Build history of the part. All positions in model axes, mm. Face numbers are marked on the shaded views. A direction names the side the tool comes from. Coordinates: 2 decimals unless noted, no trailing zeros. Order: outer loops, then holes, each group sorted by start corner. A loop starts at its lowest first (then second) coordinate and runs counter-clockwise, first axis right, second up. Notation, with made-up numbers: (69, 33) - (83, 33) arc R9 cw to (83, 42) - close; hole circle Ø10 at (8, 79). An arc over 180 degrees is marked (long way). Return JSON: item names as keys, results as strings.
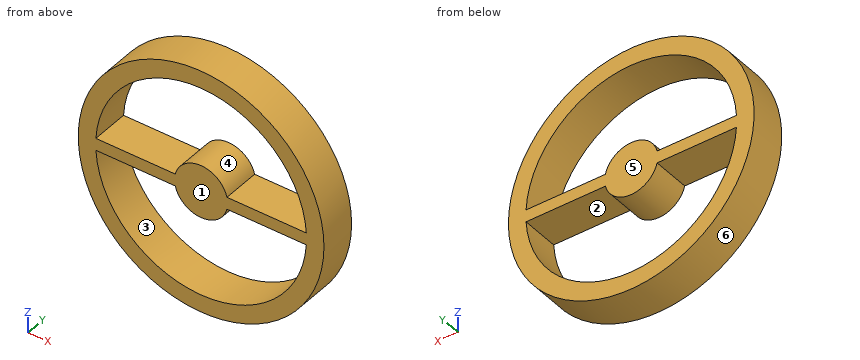
from build123d import *

# Parameters (mm, degrees)
F0_R     = 10.3601879012
F1_DEPTH = 3.175
F2_R     = 10.3601879012
F3_DEPTH = 3.175


with BuildPart() as f1:
    # F0 (on Front) → F1 (new body)
    with BuildSketch(Plane.XZ):
        Circle(F0_R)
        with BuildLine():
            ThreePointArc((9.5114533333, 0.5078193457), (9.521612731, 0.254), (9.525, 0))
            ThreePointArc((9.525, 0), (9.5215246826, -0.2572794566), (9.5111012664, -0.5143711699))
            ThreePointArc((9.5111012664, -0.5143711699), (0, -9.525), (-9.5111012664, -0.5143711699))
            ThreePointArc((-9.5111012664, -0.5143711699), (-9.524999435, -0.0032806383), (-9.5114533333, 0.5078193457))
            ThreePointArc((-9.5114533333, 0.5078193457), (0, 9.525), (9.5114533333, 0.5078193457))
        make_face(mode=Mode.SUBTRACT)
        with BuildLine():
            Line((-2.1784585047, 0.5078193457), (-9.5114533333, 0.5078193457))
            ThreePointArc((-9.5114533333, 0.5078193457), (-9.524999435, -0.0032806383), (-9.5111012664, -0.5143711699))
            Line((-9.5111012664, -0.5143711699), (-2.1769208171, -0.5143711699))
            ThreePointArc((-2.1769208171, -0.5143711699), (-2.2368617797, -0.0033649251), (-2.1784585047, 0.5078193457))
        make_face()
        with BuildLine():
            ThreePointArc((2.2368643107, 0), (2.222214889, 0.2555835118), (2.1784585047, 0.5078193457))
            ThreePointArc((2.1784585047, 0.5078193457), (0, 2.2368643107), (-2.1784585047, 0.5078193457))
            ThreePointArc((-2.1784585047, 0.5078193457), (-2.2368617797, -0.0033649251), (-2.1769208171, -0.5143711699))
            ThreePointArc((-2.1769208171, -0.5143711699), (0, -2.2368643107), (2.1769208171, -0.5143711699))
            ThreePointArc((2.1769208171, -0.5143711699), (2.2218278992, -0.2589261105), (2.2368643107, 0))
        make_face()
        with BuildLine():
            ThreePointArc((9.5111012664, -0.5143711699), (9.5215246826, -0.2572794566), (9.525, 0))
            ThreePointArc((9.525, 0), (9.521612731, 0.254), (9.5114533333, 0.5078193457))
            Line((9.5114533333, 0.5078193457), (2.1784585047, 0.5078193457))
            ThreePointArc((2.1784585047, 0.5078193457), (2.222214889, 0.2555835118), (2.2368643107, 0))
            ThreePointArc((2.2368643107, 0), (2.2218278992, -0.2589261105), (2.1769208171, -0.5143711699))
            Line((2.1769208171, -0.5143711699), (9.5111012664, -0.5143711699))
        make_face()
    extrude(amount=F1_DEPTH)

    # F2 (on face) → F3 (join)
    with BuildSketch(Plane.XZ.offset(3.175)):
        Circle(F2_R)
        with BuildLine():
            ThreePointArc((8.8731253784, 0.5078193457), (8.8840143878, 0.2540134389), (8.8876450463, 0))
            ThreePointArc((8.8876450463, 0), (8.8839199998, -0.2572934234), (8.872747983, -0.5143711699))
            Line((8.872747983, -0.5143711699), (9.5111012664, -0.5143711699))
            ThreePointArc((9.5111012664, -0.5143711699), (0, -9.525), (-9.5111012664, -0.5143711699))
            Line((-9.5111012664, -0.5143711699), (-8.872747983, -0.5143711699))
            ThreePointArc((-8.872747983, -0.5143711699), (-8.8876444406, -0.0032813423), (-8.8731253784, 0.5078193457))
            Line((-8.8731253784, 0.5078193457), (-9.5114533333, 0.5078193457))
            ThreePointArc((-9.5114533333, 0.5078193457), (0, 9.525), (9.5114533333, 0.5078193457))
            Line((9.5114533333, 0.5078193457), (8.8731253784, 0.5078193457))
        make_face(mode=Mode.SUBTRACT)
        with BuildLine():
            ThreePointArc((-8.8731253784, 0.5078193457), (0, 8.8876450463), (8.8731253784, 0.5078193457))
            Line((8.8731253784, 0.5078193457), (9.5114533333, 0.5078193457))
            ThreePointArc((9.5114533333, 0.5078193457), (0, 9.525), (-9.5114533333, 0.5078193457))
            Line((-9.5114533333, 0.5078193457), (-8.8731253784, 0.5078193457))
        make_face()
        with BuildLine():
            Line((9.5111012664, -0.5143711699), (8.872747983, -0.5143711699))
            ThreePointArc((8.872747983, -0.5143711699), (0, -8.8876450463), (-8.872747983, -0.5143711699))
            Line((-8.872747983, -0.5143711699), (-9.5111012664, -0.5143711699))
            ThreePointArc((-9.5111012664, -0.5143711699), (0, -9.525), (9.5111012664, -0.5143711699))
        make_face()
    extrude(amount=-F3_DEPTH)


solid = f1.part
1. Cut at A-A on x = 0. Give the cut face in (y, z) (3 decimals).
Check values:
{"outline": "(-3.175, -10.36) - (0, -10.36) - (0, -8.888) - (-3.175, -8.888) - close; (-3.175, -2.237) - (0, -2.237) - (0, 2.237) - (-3.175, 2.237) - close; (-3.175, 8.888) - (0, 8.888) - (0, 10.36) - (-3.175, 10.36) - close"}
2. Drop flat-ended pins along their axis: pin 1 (1.6 mm diameter, centred on x = -4.5, y = -2, fed in from +Z); pin 2 (1.5 mm diameter, centred on y = -3, z = 2.5, fed in from +X); pin 3 (2 mm diameter, centred on x = -2.5, z = 1.5, fed in from +Y); pin 4 (1 mm diameter, centred on x = 6, y = -2, fed in from -Z). Give the stop position or say it passes through.
Check values:
{"pin 1": "z = 9.68", "pin 2": "x = 10.21", "pin 3": "y = 0", "pin 4": "z = -8.78"}
3. Tool access for the marked faces 1 and 2: list every direction of +Z, -Z, +X, -X, +Y, -Y with a clear straight run to the whole face (end or side of a thin tool).
Check values:
{"face 1": "+Z, -Z, +X, -X, -Y", "face 2": "+Y, -Y"}
4. Cut at C-C on z = -4.75. Give the cut face in (x, y) (3 decimals).
Check values:
{"outline": "(-9.207, -3.175) - (-7.512, -3.175) - (-7.512, 0) - (-9.207, 0) - close; (7.512, -3.175) - (9.207, -3.175) - (9.207, 0) - (7.512, 0) - close"}
5. Cut at D-D on z = 3.5. Give the cut face in (x, y) (3 decimals), plus the area to 3 significant figures.
Check values:
{"outline": "(-9.751, -3.175) - (-8.169, -3.175) - (-8.169, 0) - (-9.751, 0) - close; (8.169, -3.175) - (9.751, -3.175) - (9.751, 0) - (8.169, 0) - close", "area": "10.0 mm²"}
6. Probe L1, parallel to Z at x = -5.25, y = -0.85; L2, parallel to X at y = -0.25, z = 1; L3, parallel to Z at x = -2.75, y = -1.4. List the from-to ranges inside material, lowest first.
Check values:
{"L1": "-8.93 to -7.17, -0.51 to 0.51, 7.17 to 8.93", "L2": "-10.31 to -8.83, -2 to 2, 8.83 to 10.31", "L3": "-9.99 to -8.45, -0.51 to 0.51, 8.45 to 9.99"}
7. Mould opens along Z. For the marked faces 3, 4, 5 and 6 say: pulls with the +Z half, pulls with the -Z half, needs draft (parallel to the pull), parting line crosses it, or undercut.
Check values:
{"face 3": "undercut", "face 4": "undercut", "face 5": "needs draft", "face 6": "parting line crosses it"}
